Can you work these out from the model? Positions are in its coordinate system, mm. A direction names the side the tool comes from. Round coordinates to 2 decimals unless told otherwise and drop trailing zeros. Write each loop counter-clockwise with the first axis right and the second up, starting at its lowest first coordinate (ties: lowest second). Pieces come first, ordered by that corner, then holes. Notation, with made-up numbers: (-6.75, -12) - (49.25, -12) arc R32 ccw to (49.25, 15) - close; hole circle Ø11 at (89, -39). An arc over 180 degrees is marked (long way). One line per item, written item: value. Start each with the question number.
(1) I want a section at C-C on x = -82. List the corners of the cut face in (y, z) for me.
(2) If I drill on L1, parallel to X at y = -138, z = -57 (1 decimal); L2, parallel to Y at x = -49.5, z = -177, over which ranges is the centre line in solid material (lowest first)? Write a range as from..to.
(3) I'm going to push flat-ended pins straight in: pin 1 Ø3 at (x, z) = (-110.5, -32) entering from +Y; pin 2 Ø16.5 at (x, y) = (-139.5, -184) entering from -Z; pin 3 Ø1.5 at (y, z) = (-92, -149) entering from +X (3 decimals); pin 4 Ø8 at (x, z) = (0.5, -152.5) entering from -Y. Where does each tip first touch, or does it pass through?
(4) On a 3-axis mill with a long thin cutter (end or side, diameter ignored), from which of +Z, -Z, +X, -X, +Y, -Y can I reach the whole of each face in a straight line? I mean faces 1 (the face through (-1, -139, -7.938)), 2 (the face through (132, -7.938, -140)), 3 (the face through (-133, -139, -7.938)). Say none if no direction works.
(5) Thinking about a two-plate mould opening in X: for faces 4 (the face through (-96.838, -110, -114)), 5 (the face through (-100.86, -161.94, -159.21)), 6 (the face through (104.775, -110, -114)), 7 (the face through (-1, -7.938, -140)), which applies, +X half, -X half, draft (parallel to the pull), parting line (faces both ways), or undercut?
(6) I want a section at B-B on z = -38. List the corners of the cut face in (x, y) for me (1 decimal), plus the area to 3 significant figures.
(7) I want a section at A-A on y = -37. List the corners of the cut face in (x, z) for me (1 decimal).
from build123d import *

# Parameters (mm, degrees)
F0_W     = 320.675
F0_H     = 275.60016
F1_DEPTH = 7.9375
F4_DEPTH = 266.7
F6_DEPTH = 265.1135
F8_R     = 6.35


with BuildPart() as f1:
    # F0 (on Front) → F1 (new body)
    with BuildSketch(Plane.XZ):
        with Locations((0, -137.80008)):
            Rectangle(F0_W, F0_H)
    extrude(amount=F1_DEPTH)

    # F3 (on face) → F4 (join)
    with BuildSketch(Plane.XZ.offset(7.9375)):
        Polygon((160.3375, 0), (-160.3375, 0), (-160.3375, -7.9375), (-104.775, -7.9375), (-104.775, -275.60016), (-96.8375, -275.60016), (-96.8375, -7.9375), (96.8375, -7.9375), (96.8375, -275.60016), (104.775, -275.60016), (104.775, -7.9375), (160.3375, -7.9375), align=None)
    extrude(amount=F4_DEPTH)

    # F5 (on face) → F6 (cut, through all)
    with BuildSketch(Plane(origin=(-104.775, 0, 0), x_dir=(0, -1, 0), z_dir=(-1, 0, 0))):
        Polygon((274.6375, -46.0375), (46.0375, -275.60016), (274.6375, -275.60016), align=None)
    extrude(amount=-F6_DEPTH, mode=Mode.SUBTRACT)

    # F8
    f8_edges = [f1.edges().sort_by_distance(p)[0] for p in [
        (-160.3375, -274.6375, -3.96875),
        (160.3375, -274.6375, -3.96875),
    ]]
    fillet(f8_edges, radius=F8_R)


solid = f1.part
Established:
1. outline: (-274.64, -7.94) - (-7.94, -7.94) - (-7.94, -275.6) - (0, -275.6) - (0, 0) - (-274.64, 0) - close
2. L1: -104.8..-96.8, 96.8..104.8
2. L2: -7.94..0
3. pin 1: y = 0
3. pin 2: z = -7.94
3. pin 3: x = 104.775
3. pin 4: y = -7.94
4. face 1: -Z, -Y
4. face 2: -Z, +X, -Y
4. face 3: -Z, -X, -Y
5. face 4: undercut
5. face 5: draft
5. face 6: +X half
5. face 7: undercut
6. outline: (-160.3, -7.9) - (-104.8, -7.9) - (-104.8, -274.6) - (-96.8, -274.6) - (-96.8, -7.9) - (96.8, -7.9) - (96.8, -274.6) - (104.8, -274.6) - (104.8, -7.9) - (160.3, -7.9) - (160.3, 0) - (-160.3, 0) - close
6. area: 6,780 mm2
7. outline: (-160.3, -7.9) - (-104.8, -7.9) - (-104.8, -275.6) - (-96.8, -275.6) - (-96.8, -7.9) - (96.8, -7.9) - (96.8, -275.6) - (104.8, -275.6) - (104.8, -7.9) - (160.3, -7.9) - (160.3, 0) - (-160.3, 0) - close
